Could you check a few things on this model? Use its own coordinates, in mm. A direction names the side the tool comes from. Give positions to 0.01 mm unless a question says otherwise; leave off trailing zeros. Loops run counter-clockwise (first coordinate to the right, second up) from the corner with the lowest first, then second, coordinate; pieces in that order, holes last. Notation, with made-up numbers: (59, -37) - (67, -37) arc R21 ccw to (67, -19) - close; hole circle Ø3 at (18.25, 44). An arc over 180 degrees is marked (long way). Use CSV: the item, a comma, the result in double quotes.
Autodesk Inventor part; units mm, degrees
ref_plane "Work Plane1" through (0, 48.05, 0) normal (0, -1, 0) x (1, 0, 0)
ref_plane "YZ Plane" through (0, 0, 0) normal (1, 0, 0) x (0, 1, 0)
ref_plane "XZ Plane" through (0, 0, 0) normal (0, 1, 0) x (-1, 0, 0)
sketch "Sketch1" plane through (0, 0, 0) normal (0, 1, 0) x (-1, 0, 0)
  line L0 (0, 0) -> (-7.5, 0)
  line L1 (-7.5, -15) -> (0, -15)
  line L2 (0, -15) -> (0, 0)
  line L3 (-7.5, -9.5) -> (-9.5, -9.5)
  line L4 (-9.5, -9.5) -> (-9.5, -5.5)
  line L5 (-9.5, -5.5) -> (-7.5, -5.5)
  line L6 (-7.5, 0) -> (-7.5, -5.5)
  line L7 (-7.5, -9.5) -> (-7.5, -15)
  line L8 (-7.6, -15.1) -> (0.1, -15.1)
  line L9 (0.1, -15.1) -> (0.1, 0.1)
  line L10 (0.1, 0.1) -> (-7.6, 0.1)
  line L11 (-7.6, 0.1) -> (-7.6, -5.4)
  line L12 (-7.6, -5.4) -> (-9.6, -5.4)
  line L13 (-9.6, -5.4) -> (-9.6, -9.6)
  line L14 (-9.6, -9.6) -> (-7.6, -9.6)
  line L15 (-7.6, -9.6) -> (-7.6, -15.1)
  line L16 (0, 0) -> (-12.1, 0)
  line L17 (-12.1, 0) -> (-12.1, -19.6)
  line L18 (-12.1, -19.6) -> (0, -19.6)
  line L19 (0, -19.6) -> (0, 0)
  point P0 (-7.6, 0)
  point P1 (0, -15.1)
  dimension "d2" = 7.5
  dimension "d3" = 15
  dimension "d8" = 4
  dimension "d9" = 2
  dimension "d10" = 5.5
  dimension "d11" = 0.1
  dimension "d12" = 4.5
  dimension "d13" = 4.5
extrude "Extrusion1" add sketch "Sketch1" along normal blind 96.1 contours L11 L12 L13 L14 L15 L8 L19 L18 L17 L16
ref_plane "Work Plane1" through (0, 48.05, 0) normal (0, -1, 0) x (1, 0, 0)
sketch "Sketch2" plane through (0, 96.1, 0) normal (0, 1, 0) x (1, 0, 0)
  line L0 (7.6, 9.6) -> (9.6, 9.6)
  line L1 (9.6, 9.6) -> (9.6, 5.4)
  line L2 (9.6, 5.4) -> (7.6, 5.4)
  line L3 (7.6, 5.4) -> (7.6, 0)
  line L4 (7.6, 0) -> (12.1, 0)
  line L5 (12.1, 0) -> (12.1, 19.6)
  line L6 (12.1, 19.6) -> (0, 19.6)
  line L7 (0, 19.6) -> (0, 15.1)
  line L8 (0, 15.1) -> (7.6, 15.1)
  line L9 (7.6, 15.1) -> (7.6, 9.6)
  line L10 (12.1, 0) -> (12.1, 19.6)
  line L11 (12.1, 19.6) -> (0, 19.6)
  line L12 (0, 19.6) -> (0, 0)
  line L13 (0, 0) -> (12.1, 0)
  line L14 (12.1, 0) -> (12.1, 19.6)
  circle A0 centre (0, 7.5) radius 2.75
  line L15 (0, 7.5) -> (9.6, 7.5)
  line L16 (9.6, 9.6) -> (9.6, 5.4)
  point P0 (0, 10.25)
  point P1 (0, 4.75)
  dimension "d16" = 5.5
extrude "Extrusion2" add sketch "Sketch2" along normal blind 3.9 contours L9 L8 L7 L6 L5 L4 L3 L2 L1 L0 | L0 L1 L15 A0 L12 L8 L9 | L1 L2 L3 L13 L12 A0 L15
mirror "Mirror1" about plane through (0, 48.05, 0) normal (0, -1, 0) of "Extrusion2"
chamfer "Chamfer1" distance 1 angle 45 2 edges at (2.75, 96.1, -7.5) (2.75, -3.9, -7.5)
sketch "Sketch5" plane through (12.1, 100, -19.6) normal (0, 0, -1) x (-1, 0, 0)
  circle A0 centre (12.1, -95.4279) radius 3.275
  line L0 (12.1, -88.9558) -> (17.705, -92.1919)
  line L1 (17.705, -92.1919) -> (17.705, -98.664)
  line L2 (17.705, -98.664) -> (12.1, -101.9)
  line L3 (12.1, -101.9) -> (6.495, -98.664)
  line L4 (6.495, -98.664) -> (6.495, -92.1919)
  line L5 (6.495, -92.1919) -> (12.1, -88.9558)
  line L6 (6.495, -92.1919) -> (17.705, -98.664) construction
  line L7 (17.705, -92.1919) -> (6.495, -98.664) construction
  line L8 (12.1, -103.9) -> (12.1, 0)
  dimension "d26" = 6.55
  dimension "d27" = 11.21
  dimension "d48" = 2
extrude "Extrusion3" cut sketch "Sketch5" against normal blind 2
extrude "Extrusion7" cut sketch "Sketch5" against normal through all contours A0 L8 | L8 A0
sketch "Sketch7" plane through (12.1, 100, -19.6) normal (0, 0, -1) x (-1, 0, 0)
  line L0 (0, -103.9) -> (0, 0)
  line L1 (12.1, -86.9558) -> (0, -86.9558)
  line L2 (0, -86.9558) -> (0, -103.9)
  line L3 (0, -103.9) -> (12.1, -103.9)
  line L4 (12.1, -103.9) -> (12.1, -86.9558)
  arc A0 (12.1, -92.1529) -> (12.1, -98.7029) centre (12.1, -95.4279) ccw
  line L5 (12.1, -88.9558) -> (12.1, -92.1529)
  line L6 (6.495, -92.1919) -> (12.1, -88.9558)
  line L7 (6.495, -98.664) -> (6.495, -92.1919)
  line L8 (12.1, -101.9) -> (6.495, -98.664)
  line L9 (12.1, -98.7029) -> (12.1, -101.9)
  line L10 (12.1, -88.9558) -> (12.1, 0)
  point P0 (12.1, -100)
  point P1 (12.1, -88.9558)
  point P2 (0, -86.9558)
  dimension "d51" = 2
extrude "Extrusion8" add sketch "Sketch7" along normal blind 2 contours L0 L1 L4 L6 L7 L8 L3
chamfer "Chamfer4" distance 2 angle 45 1 edges at (6.05, 13.0442, -19.6)
chamfer "Chamfer3" distance 1 angle 45 10 edges at (6.05, -3.9, 0) (12.1, 100, -9.8) (6.05, 100, -19.6) (6.05, 100, 0) (12.1, 48.05, 0) (12.1, -3.9, -10.8) (6.05, -3.9, -21.6) (12.1, 14.0441, -20.5999) (12.1, 57.522, -19.6) (12.1, 4.5721, -21.6)
properties part number "lead_screw_housing"
1) Suppose I cut it at C-C (x = 1). State how many separate pieces and enclosed holes the cut face has, plus the area to 3 significant figures.
Answer below:
separate pieces,"4"
enclosed holes,"0"
area,"514 mm2"
2) I'm going to push flat-ended pins straight in: P1, Ø6, axis at x = 3.5, y = 49.5, coming from the +Z side; P2, Ø6, axis at y = 49.5, z = -11.5, coming from the -X side; P3, Ø3.5, axis at y = 67.5, z = -7.5, coming from the -X side. Where does each tip first touch, or does it pass through?
Answer below:
P1,"stops at z = -15.1"
P2,"stops at x = 7.6"
P3,"stops at x = 9.6"
3) We'd pull the mould along Y, two halves only. Please class faces 5 (the flat face through (7.6, 47, -12)), 6 (the flat face through (6, -3.9, -11)), 7 (the flat face through (7, 5, -21.6)): +Y half, -Y half, draft (parallel to the pull), parting line (faces both ways), or undercut.
Answer below:
face 5,"undercut"
face 6,"-Y half"
face 7,"draft"
4) I need wall thicknesses on line 1 along Z through (x, y) = (8.25, 51); line 2 along Y through (x, z) = (5.5, -18.25); line 3 along Y through (x, z) = (7, -12.75). Which ranges of each line are inside material? Lowest first, please.
Answer below:
line 1,"z = -19.6 to -9.6, -5.4 to 0"
line 2,"y = -3.9 to 1.28, 7.87 to 100"
line 3,"y = -3.9 to 0, 96.1 to 100"
5) Which directions (+Z, -Z, +X, -X, +Y, -Y) give clear straight access to the entire face, cutting with the end or side of a thin tool? Please do faces 1 (the flat face through (9.6, 47, -7)), 2 (the flat face through (0, -2, -16)), 3 (the flat face through (4, 47, -15.1)), 4 (the flat face through (3.5, 4.7, -17.6)).
Answer below:
face 1,"-X"
face 2,"+Z, -Z, -X, +Y, -Y"
face 3,"+Z, -X"
face 4,"-Z, -X"
6) Suppose I cut it at A-A (y = 37). Please give me the cut outline in (x, z), plus the area to 3 significant figures.
Answer below:
outline,"(0, -19.6) - (11.1, -19.6) - (12.1, -18.6) - (12.1, -1) - (11.1, 0) - (7.6, 0) - (7.6, -5.4) - (9.6, -5.4) - (9.6, -9.6) - (7.6, -9.6) - (7.6, -15.1) - (0, -15.1) - close"
area,"113 mm2"
7) Suppose I cut it at B-B (z = -7.5). Please give me the cut outline in (x, y).
Answer below:
outline,"(2.75, -2.9) - (3.75, -3.9) - (11.1, -3.9) - (12.1, -2.9) - (12.1, 99) - (11.1, 100) - (2.75, 100) - (2.75, 97.1) - (3.75, 96.1) - (9.6, 96.1) - (9.6, 0) - (2.75, 0) - close"
